The model under review builds one solid part; all positions refer to its coordinate system, in mm. A direction names the side the tool comes from. Round coordinates to 2 decimals unless told otherwise and drop trailing zeros. Order: outer loops, then holes, each group sorted by start corner. A loop starts at its lowest first (then second) coordinate and runs counter-clockwise, first axis right, second up. Notation, with made-up numbers: M 23,86 L 36,86 A17 ccw 36,118 Z; hole C 45,33.5 d3. An arc over 180 degrees is marked long. Answer as a JSON object with one key per item and string values. Group by question number.
1. Clearance check with flat-ended pins moving along their axes: P1, Ø4, axis at x = 8, z = 8, coming from the -Y side; P2, Ø9.5, axis at x = 59.509, y = 0, coming from the -Z side; P3, Ø5.5, axis at x = -12.08, y = 31.25, coming from the -Z side; P4, Ø1, axis at x = 22, z = 8, coming from the +Y side. State where each tip first meets the part, or that it passes through.
2. Mouldability with a two-part tool opening along Y and no side actions: class faces 1 (the face through (58, -39, 0)), 2 (the face through (4.397, 33.408, 2.437)) as released by +Y, released by -Y, zero draft, split by the parting line, or undercut.
3. Add section A-A on y = 0. State the section outline as (x, z) points.
4. To check wall thickness, follow probe 1 along X at (y, z) = (0, 7.75); probe 2 along Y at (x, z) = (66, 2.5); probe 3 along X at (y, z) = (10, 5.75). State the ranges of each line that lie inside material, in increasing order. Write a range as [from, to].
5. Machinability: for faces 3 (the face through (53, 0, 0)), 4 (the face through (55, -5, 3)), 5 (the face through (75.494, 0.703, 3.204)), which of the approach directions +Z, -Z, +X, -X, +Y, -Y give a long, thin tool a straight path to every point of the face, cutting with its end or side? Answer none if there is none.
6. Add section B-B on y = 31.25. Give the number of separate pieces and of enclosed holes in the cut face, and give its area (3 significant figures).
7. Add section D-D on x = 13. State the section outline as (y, z) points, and give its area (3 significant figures).
Autodesk Inventor part; units mm, degrees
ref_plane "YZ Plane" through (0, 0, 0) normal (1, 0, 0) x (0, 1, 0)
ref_plane "XZ Plane" through (0, 0, 0) normal (0, 1, 0) x (-1, 0, 0)
ref_plane "XY Plane" through (0, 0, 0) normal (0, 0, 1) x (1, 0, 0)
sketch "Sketch1" plane through (0, 0, 0) normal (0, 0, 1) x (1, 0, 0)
  circle A0 centre (-11.3135, -11.3135) radius 2
  circle A1 centre (-11.3135, 11.3135) radius 2
  circle A2 centre (11.3135, 11.3135) radius 2
  circle A3 centre (11.3135, -11.3135) radius 2
  circle A4 centre (-15.3135, 11.3135) radius 2
  circle A5 centre (-7.3135, 11.3135) radius 2
  circle A6 centre (7.3135, 11.3135) radius 2
  circle A7 centre (15.3135, 11.3135) radius 2
  circle A8 centre (15.3135, -11.3135) radius 2
  circle A9 centre (7.3135, -11.3135) radius 2
  circle A10 centre (-7.3135, -11.3135) radius 2
  circle A11 centre (-15.3135, -11.3135) radius 2
  line L0 (-15.3135, 13.3135) -> (-7.3135, 13.3135)
  line L1 (-7.3135, 9.3135) -> (-15.3135, 9.3135)
  line L2 (-15.3135, -9.3135) -> (-7.3135, -9.3135)
  line L3 (-7.3135, -13.3135) -> (-15.3135, -13.3135)
  line L4 (7.3135, -9.3135) -> (15.3135, -9.3135)
  line L5 (15.3135, -13.3135) -> (7.3135, -13.3135)
  line L6 (15.3135, 9.3135) -> (7.3135, 9.3135)
  line L7 (15.3135, 13.3135) -> (7.3135, 13.3135)
  circle A12 centre (0, 0) radius 8.25
  circle A13 centre (5, 0) radius 8.25
  circle A14 centre (-5, 0) radius 8.25
  line L8 (-5, 8.25) -> (5, 8.25)
  line L9 (5, -8.25) -> (-5, -8.25)
  circle A15 centre (0, 0) radius 42.5
  circle A16 centre (59.509, 0) radius 50.7821
  line L10 (-5.9149, 42.0864) -> (52.4415, 50.2878)
  line L11 (-5.9149, -42.0864) -> (52.4415, -50.2878)
  line L12 (-13.25, 0) -> (13.25, 0)
  circle A17 centre (59.509, 0) radius 11
  arc A18 (-5.9149, 42.0864) -> (-5.9149, -42.0864) centre (0, 0) ccw
  line L13 (-42.5, 0) -> (156.5802, 0)
  circle A19 centre (59.509, 0) radius 90
  point P0 (-3.1314, -32.3793)
  point P1 (23.2633, -35.5678)
  point P2 (23.2633, 35.5678)
  point P3 (-2.5, -7.8621)
  point P4 (0, -8.25)
  dimension "d0" = 4
  dimension "d1" = 22.627
  dimension "d2" = 22.627
  dimension "d3" = 11.3135
  dimension "d4" = 11.3135
  dimension "d5" = 4
  dimension "d6" = 4
  dimension "d7" = 4
  dimension "d8" = 4
  dimension "d9" = 4
  dimension "d10" = 4
  dimension "d11" = 4
  dimension "d12" = 4
  dimension "d15" = 16.5
  dimension "d16" = 5
  dimension "d17" = 5
  dimension "d18" = 85
  dimension "d19" = 8
  dimension "d20" = 59.509
  dimension "d21" = 22
  dimension "d24" = 85
  dimension "d116" = 180
extrude "Extrusion1" add sketch "Sketch1" along normal blind 10 contours A0 | A10 L3 A0 | A0 L2 A10 | A10 | A0 A11 L2 | L3 A11 A0 | A11 | A1 | A5 L1 A1 | A1 L0 A5 | A5 | A1 A4 L0 | L1 A4 A1 | A4 | A2 A16 | A7 L6 A2 | A2 L7 A7 | A7 | L7 A16 A15 L13 A13 L6 A7 | A2 A16 L7 | L6 A16 A2 | A16 A2 | A2 A6 L7 A16 | L7 A6 L6 A16 A13 L8 A14 L13 A19 A15 | A16 L6 A6 A2 | A6 | A16 L13 A17 A15 | A15 L10 A16 | A16 L12 A12 A13 | A13 L12 A16 | L13 A17 A16 A15 | A15 A16 L5 A8 L4 A13 L13 | A15 A19 L13 A16 L10 | A13 A16 L12 | A13 A12 L8 | A16 A13 A12 L12 | A16 L11 A15 | A15 A19 L13 A14 L9 A13 A16 L4 A9 L5 | L13 A19 A15 L11 A16 | A13 A14 A12 | A12 L12 A14 A13 | A12 A14 L8 | A12 A13 A14 L12 | A16 A3 L5 | L5 A9 A3 A16 | L9 A12 A13 | A16 A3 A9 L4 | L4 A3 A16 | A14 L12 A13 | A13 L12 A12 A14 | A12 L12 A14 | A12 A14 A13 | A14 A13 L12 | A3 A16 | A3 A8 L5 | A9 | A3 A16 | L12 A12 A14 | L9 A14 A12 | L4 A8 A3 | A13 A14 A12 L12 | A8
sketch "Sketch18" plane through (59.509, 0, 0) normal (0, 0, -1) x (-1, 0, 0)
  circle A0 centre (0, 0) radius 35
  circle A1 centre (0, 0) radius 90
  circle A2 centre (0, 0) radius 11
  circle A3 centre (0, 0) radius 16
  point P0 (59.509, 0)
  dimension "d127" = 70
  dimension "d130" = 5
extrude "Extrusion9" cut sketch "Sketch18" against normal blind 6.5 contours A0 | A2
sketch "Sketch20" plane through (59.509, 0, 0) normal (0, 0, -1) x (-1, 0, 0)
  circle A0 centre (0, 0) radius 11
  circle A1 centre (0, 0) radius 11
  circle A2 centre (0, 0) radius 6
  point P0 (59.509, 0)
  dimension "d136" = 12
extrude "Extrusion11" add sketch "Sketch20" against normal blind 3
sketch "Sketch22" plane through (59.509, 0, 0) normal (0, 0, -1) x (-1, 0, 0)
  circle A0 centre (55.7915, 31.25) radius 1.621
  circle A1 centre (71.5915, 31.25) radius 1.621
  circle A2 centre (71.5915, -31.2504) radius 1.621
  circle A3 centre (55.7915, -31.2504) radius 1.621
  circle A4 centre (71.5915, -31.2504) radius 1.621
  circle A5 centre (55.7915, -31.2504) radius 1.621
  circle A6 centre (71.5915, 31.25) radius 1.621
  circle A7 centre (55.7915, 31.25) radius 1.621
  point P0 (59.509, 0)
hole "Hole4" at (-12.0825, 31.25, 0) at (3.7175, 31.25, 0) at (-12.0825, -31.2504, 0) at (3.7175, -31.2504, 0) direction (0, 0, 1) diameter 4.2 end through all countersink diameter 9.4 countersink angle 90
sketch "Sketch23" plane through (59.509, 0, 0) normal (0, 0, -1) x (-1, 0, 0)
  circle A0 centre (-26.526, -31.25) radius 2.4585
  circle A1 centre (26.526, -31.25) radius 2.4585
  circle A2 centre (-26.526, 31.25) radius 1.621
  circle A3 centre (26.526, 31.25) radius 1.621
  circle A4 centre (26.526, -31.25) radius 2.4585
  circle A5 centre (26.526, 31.25) radius 1.621
  circle A6 centre (-26.526, -31.25) radius 2.4585
  circle A7 centre (0, 0) radius 90
  circle A8 centre (0, 0) radius 11
  circle A9 centre (-26.526, 31.25) radius 1.621
  point P0 (59.509, 0)
hole "Hole5" at (86.035, 31.25, 0) at (86.035, -31.25, 0) at (32.983, -31.25, 0) at (32.983, 31.25, 0) direction (0, 0, 1) diameter 4.5 depth 14.2 tip angle 118 countersink diameter 9.4 countersink angle 90
equation "\"d2\" = d1"
equation "\"d5\" = d0"
equation "\"d6\" = d5"
equation "\"d7\" = d6"
equation "\"d8\" = d7"
equation "\"d9\" = d5"
equation "\"d10\" = d9"
equation "\"d11\" = d10"
equation "\"d12\" = d11"
equation "\"d17\" = d16"
properties part number "base bovenkant 10 mm" material "Aluminum 6061"
Recorded:
{
 "1": {"P1": "stops at y = -75.16", "P2": "passes through", "P3": "stops at z = 1.95", "P4": "stops at y = 82.04"},
 "2": {"face 1": "zero draft", "face 2": "undercut"},
 "3": {"outline": "M -30.49,0 L 24.51,0 L 24.51,6.5 L 43.51,6.5 L 43.51,0 L 53.51,0 L 53.51,3 L 48.51,3 L 48.51,10 L -30.49,10 Z; M 65.51,0 L 75.51,0 L 75.51,6.5 L 94.51,6.5 L 94.51,0 L 149.51,0 L 149.51,10 L 70.51,10 L 70.51,3 L 65.51,3 Z"},
 "4": {"probe 1": "x = [-30.49, 48.51], [70.51, 149.51]", "probe 2": "y = [-89.77, -34.39], [-14.62, 14.62], [34.39, 89.77]", "probe 3": "x = [-29.93, 25.97], [47.02, 54.93], [64.09, 72], [93.05, 148.95]"},
 "5": {"face 3": "-Z, +X, -X, +Y, -Y", "face 4": "+Z", "face 5": "-Z"},
 "6": {"separate pieces": "5", "enclosed holes": "0", "area": "1,280 mm²"},
 "7": {"outline": "M -77.05,0 L 77.05,0 L 77.05,10 L -77.05,10 Z", "area": "1,540 mm²"}
}
